Here's the drawing with two shaded views (mm, measured from the low corner). I have some questions. A direction names the side the tool comes from. Give positions to 0.01 mm unless a question says otherwise; leave off trailing zeros. Loops run counter-clockwise (first coordinate to the right, second up) from the corner with the lowest first, then second, coordinate; pieces in that order, holes last. Notation, with made-up numbers: M 9,60 L 26,60 A21 cw 26,76 Z; hole C 77,-35.5 d8. An arc over 180 degrees is marked long. Put each result on its own line as item: value. Start each with the question number.
1) For P1, Ø5, axis at x = 7, y = 13, coming from the -Z side; P2, Ø1, axis at x = 11.5, z = 12, coming from the -Y side; P3, Ø6, axis at x = 12.5, z = 2, coming from the +Y side, each with a flat end and sliding along its axis, tell me the tip position at first contact or that it passes through.
2) For the marked faces 1 and 2, which set-ups out of +Z, -Z, +X, -X, +Y, -Y let a thin tool reach every point of the face, with its end or its side?
3) Imagine slicing it at A-A (y = 7). Write out the boundary of the cut face in (x, z).
4) Please list where these lines run through material, in increasing order: line 1 along Z through (x, y) = (7.5, 3.5); line 2 along Z through (x, y) = (8.25, 2); line 3 along Y through (x, z) = (8.5, 5). Write a range as from..to.
5) If we mould it in two halves opening along X, with no side actions, what happens to the marked faces 3, 4 and 5? For each: +X half, -X half, draft (parallel to the pull), parting line (faces both ways), or undercut.
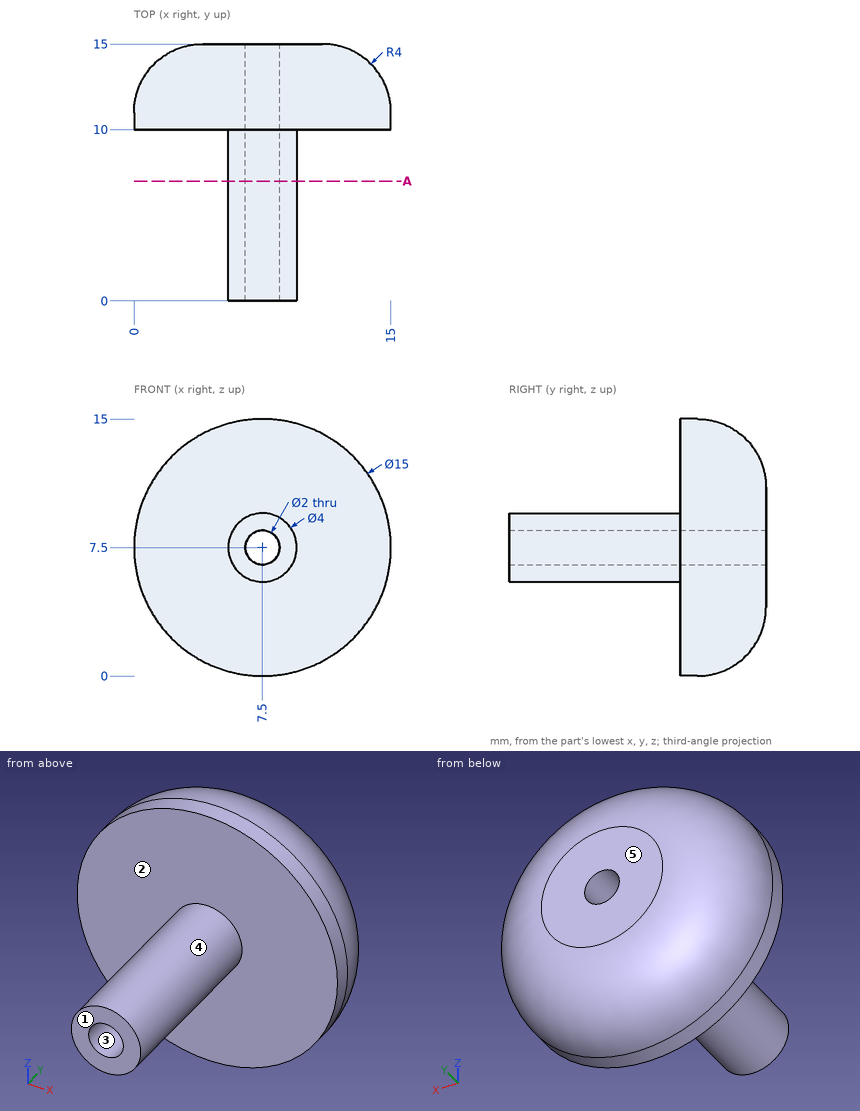
Recorded:
1. P1: z = 0
1. P2: y = 10
1. P3: y = 14.89
2. face 1: +Z, -Z, +X, -X, -Y
2. face 2: -Y
3. outline: C 7.5,7.5 d4; hole C 7.5,7.5 d2
4. line 1: 5.5..6.5, 8.5..9.5
4. line 2: 5.65..6.84, 8.16..9.35
4. line 3: 10..15
5. face 3: undercut
5. face 4: parting line
5. face 5: draft
